The model under review builds one solid part; all positions refer to its coordinate system, in mm. Give positions to 0.01 mm unless a question says otherwise; leave off trailing zeros. Loops run counter-clockwise (first coordinate to the right, second up) from the corner with the lowest first, then second, coordinate; pieces in that order, holes last. Notation, with made-up numbers: M 73,13.25 L 112,13.25 A7 ccw 112,22.25 Z; hole C 40.5,57 d4. An arc over 180 degrees is marked long. Write item = value, one per line. Start each with the question number.
1. We need section B-B on z = 1.5. Count the separate pieces of the cut face and the enclosed holes in it, then the cut area to 3 significant figures.
2. For pin 1 (1.5 mm diameter, centred on x = 66.5, z = 1, fed in from +Y); pin 2 (1.5 mm diameter, centred on y = -84.5, z = 1.5, fed in from +X); pin 3 (0.9 mm diameter, centred on y = 43.5, z = 1, fed in from +X), all flat-tipped, find the tip position at first contact; note any pin that passes through.
3. We need section A-A on x = -4.5. Give the boundary of the cut face in (y, z).
4. We need section C-C on x = -31.5. Give the boundary of the cut face in (y, z), then the cut area to 3 significant figures.
5. Wall thickness on line 1 along X through (y, z) = (-45.5, 1.2); line 2 along Y through (x, z) = (9, 0.35); line 3 along X through (y, z) = (-89, 1.4): over which ranges is each line inside the solid? List them lowest first. Write a range as from..to.
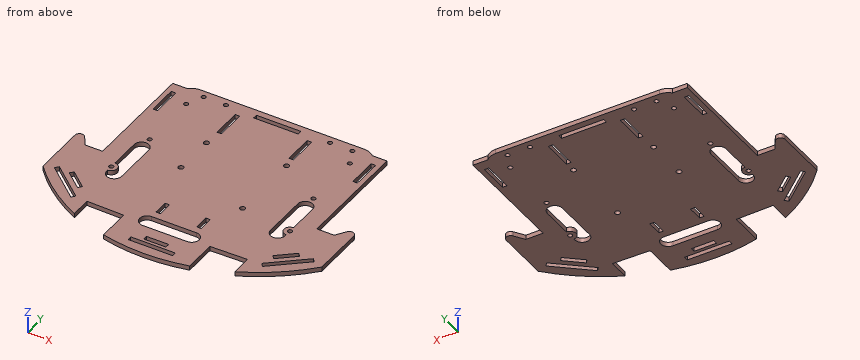
from build123d import *

# Parameters (mm, degrees)
SKETCH1_R           = 1.5
BOSS_EXTRUDE1_DEPTH = 3
SKETCH12_W          = 3
SKETCH12_H          = 20
BOSS_EXTRUDE3_DEPTH = 3
SKETCH13_W          = 3
SKETCH13_H          = 20
CUT_EXTRUDE5_DEPTH  = 3
SKETCH15_W          = 30
SKETCH15_H          = 3
BOSS_EXTRUDE4_DEPTH = 3
CUT_EXTRUDE7_DEPTH  = 3
CUT_EXTRUDE8_DEPTH  = 5
SKETCH18_R          = 1.5
SKETCH18_W          = 30
SKETCH18_H          = 3
CUT_EXTRUDE9_DEPTH  = 3
FILLET4_R           = 3
SKETCH25_R          = 1.5
CUT_EXTRUDE11_DEPTH = 10
CUT_EXTRUDE12_DEPTH = 10
SKETCH27_W          = 15
SKETCH27_H          = 3
CUT_EXTRUDE13_DEPTH = 10
SKETCH34_W          = 3
SKETCH34_H          = 10
CUT_EXTRUDE14_DEPTH = 10
SKETCH35_R          = 1.75
CUT_EXTRUDE15_DEPTH = 10


with BuildPart() as part:
    # Sketch1 → Boss-Extrude1 (new body)
    with BuildSketch(Plane.XY):
        with BuildLine():
            Line((-65, 40), (-65, -45))
            ThreePointArc((-65, -45), (-62.071067812, -52.071067812), (-55, -55))
            Line((-55, -55), (55, -55))
            ThreePointArc((55, -55), (62.071067812, -52.071067812), (65, -45))
            Line((65, -45), (65, 40))
            ThreePointArc((65, 40), (62.071067812, 47.071067812), (55, 50))
            Line((55, 50), (-55, 50))
            ThreePointArc((-55, 50), (-62.071067812, 47.071067812), (-65, 40))
        make_face()
        with Locations((-50, 45)):
            Circle(SKETCH1_R, mode=Mode.SUBTRACT)
        with Locations((50, 45)):
            Circle(SKETCH1_R, mode=Mode.SUBTRACT)
        with Locations((-60, -40)):
            Circle(SKETCH1_R, mode=Mode.SUBTRACT)
        with Locations((60, -40)):
            Circle(SKETCH1_R, mode=Mode.SUBTRACT)
    extrude(amount=BOSS_EXTRUDE1_DEPTH)

    # Sketch12 → Boss-Extrude3 (add)
    with BuildSketch(Plane(origin=(0, 0, 0), x_dir=(-1, 0, 0), z_dir=(0, 0, -1))):
        with BuildLine():
            Line((65, 40), (65, -30))
            Line((65, -30), (72, -30))
            Line((72, -30), (72, 40))
            Line((72, 40), (72, 47.071067812))
            Line((72, 47.071067812), (62.071067812, 47.071067812))
            ThreePointArc((62.071067812, 47.071067812), (64.238795325, 43.826834324), (65, 40))
        make_face()
        with Locations((67.174969976, 30)):
            Rectangle(SKETCH12_W, SKETCH12_H, mode=Mode.SUBTRACT)
        with BuildLine():
            Line((-72, 40), (-72, -30))
            Line((-72, -30), (-65, -30))
            Line((-65, -30), (-65, 40))
            ThreePointArc((-65, 40), (-64.238795325, 43.826834324), (-62.071067812, 47.071067812))
            Line((-62.071067812, 47.071067812), (-72, 47.071067812))
            Line((-72, 47.071067812), (-72, 40))
        make_face()
        with Locations((-67.174969976, 30)):
            Rectangle(SKETCH12_W, SKETCH12_H, mode=Mode.SUBTRACT)
    extrude(amount=-BOSS_EXTRUDE3_DEPTH)

    # Sketch13 → Cut-Extrude5 (cut)
    with BuildSketch(Plane(origin=(0, 0, 0), x_dir=(-1, 0, 0), z_dir=(0, 0, -1))):
        with Locations((24.174969976, 30)):
            Rectangle(SKETCH13_W, SKETCH13_H)
        with Locations((-24.174969976, 30)):
            Rectangle(SKETCH13_W, SKETCH13_H)
    extrude(amount=-CUT_EXTRUDE5_DEPTH, mode=Mode.SUBTRACT)

    # Sketch15 → Boss-Extrude4 (add)
    with BuildSketch(Plane(origin=(0, 0, 0), x_dir=(-1, 0, 0), z_dir=(0, 0, -1))):
        with BuildLine():
            Line((73.674969976, -30), (72, -30))
            Line((72, -30), (65, -30))
            Line((65, -30), (65, -45))
            ThreePointArc((65, -45), (62.071067812, -52.071067812), (55, -55))
            Line((55, -55), (-55, -55))
            ThreePointArc((-55, -55), (-62.071067812, -52.071067812), (-65, -45))
            Line((-65, -45), (-65, -30))
            Line((-65, -30), (-72, -30))
            Line((-72, -30), (-73.674969976, -30))
            Line((-73.674969976, -30), (-83.674969976, -30))
            Line((-83.674969976, -30), (-93.674969976, -15))
            Line((-93.674969976, -15), (-93.674969976, -60))
            ThreePointArc((-93.674969976, -60), (-75.11867005, -76.957696294), (-53.544667826, -89.859717787))
            Line((-53.544667826, -89.859717787), (-53.544667826, -77.921197712))
            Line((-53.544667826, -77.921197712), (-43.544667826, -77.921197712))
            Line((-43.544667826, -77.921197712), (-28.544667826, -78.447755309))
            Line((-28.544667826, -78.447755309), (-28.544667826, -98.657929362))
            ThreePointArc((-28.544667826, -98.657929362), (0.412515012, -102.058251887), (29.36969785, -98.657929362))
            Line((29.36969785, -98.657929362), (29.36969785, -78.447755309))
            Line((29.36969785, -78.447755309), (44.36969785, -77.921197712))
            Line((44.36969785, -77.921197712), (54.36969785, -77.921197712))
            Line((54.36969785, -77.921197712), (54.36969785, -89.791641118))
            ThreePointArc((54.36969785, -89.791641118), (75.506234101, -76.853587855), (93.674969976, -60))
            Line((93.674969976, -60), (93.674969976, -15))
            Line((93.674969976, -15), (83.674969976, -30))
            Line((83.674969976, -30), (73.674969976, -30))
        make_face()
        Polygon((-64.364341028, -77.265224848), (-87.294606331, -57.920899244), (-85.360173771, -55.627872713), (-62.429908467, -74.972198318), align=None, mode=Mode.SUBTRACT)
        with Locations((0, -93.735273214)):
            Rectangle(SKETCH15_W, SKETCH15_H, mode=Mode.SUBTRACT)
        Polygon((-65.960254421, -67.497898332), (-77.422828052, -57.822702946), (-75.487788974, -55.53018822), (-64.025215344, -65.205383606), align=None, mode=Mode.SUBTRACT)
        Polygon((85.360173771, -55.627872713), (87.294606331, -57.920899244), (64.364341028, -77.265224848), (62.429908467, -74.972198318), align=None, mode=Mode.SUBTRACT)
        Polygon((77.394030345, -57.788043022), (65.932380202, -67.464332393), (63.997122328, -65.172002365), (75.458772471, -55.495712994), align=None, mode=Mode.SUBTRACT)
    extrude(amount=-BOSS_EXTRUDE4_DEPTH)

    # Sketch16 → Cut-Extrude7 (cut)
    with BuildSketch(Plane(origin=(0, 0, 0), x_dir=(-1, 0, 0), z_dir=(0, 0, -1))):
        with BuildLine():
            Line((-60, -44), (-60, -45))
            ThreePointArc((-60, -45), (-55, -50), (-50, -45))
            Line((-50, -45), (-50, -15))
            ThreePointArc((-50, -15), (-55, -10), (-60, -15))
            Line((-60, -15), (-60, -36))
            ThreePointArc((-60, -36), (-56, -40), (-60, -44))
        make_face()
        with BuildLine():
            Line((60, -36), (60, -15))
            ThreePointArc((60, -15), (55, -10), (50, -15))
            Line((50, -15), (50, -45))
            ThreePointArc((50, -45), (55, -50), (60, -45))
            Line((60, -45), (60, -44))
            ThreePointArc((60, -44), (56, -40), (60, -36))
        make_face()
    extrude(amount=-CUT_EXTRUDE7_DEPTH, mode=Mode.SUBTRACT)

    # Sketch17 → Cut-Extrude8 (cut)
    with BuildSketch(Plane(origin=(0, 0, 0), x_dir=(-1, 0, 0), z_dir=(0, 0, -1))):
        with BuildLine():
            Line((-15, -69.235273214), (15, -69.235273214))
            ThreePointArc((15, -69.235273214), (20, -74.235273214), (15, -79.235273214))
            Line((15, -79.235273214), (-15, -79.235273214))
            ThreePointArc((-15, -79.235273214), (-20, -74.235273214), (-15, -69.235273214))
        make_face()
    extrude(amount=-CUT_EXTRUDE8_DEPTH, mode=Mode.SUBTRACT)

    # Sketch18 → Cut-Extrude9 (cut)
    with BuildSketch(Plane(origin=(0, 0, 0), x_dir=(-1, 0, 0), z_dir=(0, 0, -1))):
        with Locations((55, 34)):
            Circle(SKETCH18_R)
        with Locations((55, -6)):
            Circle(SKETCH18_R)
        with Locations((-55, 34)):
            Circle(SKETCH18_R)
        with Locations((-55, -6)):
            Circle(SKETCH18_R)
        with Locations((0, 44.264726786)):
            Rectangle(SKETCH18_W, SKETCH18_H)
    extrude(amount=-CUT_EXTRUDE9_DEPTH, mode=Mode.SUBTRACT)

    # Fillet4
    fillet4_edges = [part.edges().sort_by_distance(p)[0] for p in [
        (93.674969976, -15, 1.5),
        (-93.674969976, -15, 1.5),
    ]]
    fillet(fillet4_edges, radius=FILLET4_R)

    # Sketch25 → Cut-Extrude11 (cut)
    with BuildSketch(Plane.XY.offset(3)):
        with Locations((-35, 45)):
            Circle(SKETCH25_R)
        with Locations((35, 45)):
            Circle(SKETCH25_R)
    extrude(amount=-CUT_EXTRUDE11_DEPTH, mode=Mode.SUBTRACT)

    # Sketch26 → Cut-Extrude12 (cut)
    with BuildSketch(Plane.XY.offset(3)):
        Polygon((-54.36969785, -77.921197712), (-54.36969785, -75.921197712), (-29.36969785, -76.450833315), (-29.36969785, -78.447755309), align=None)
        Polygon((28.544667826, -78.447755309), (28.544667826, -76.450833315), (53.544667826, -75.921197712), (53.544667826, -77.921197712), align=None)
    extrude(amount=-CUT_EXTRUDE12_DEPTH, mode=Mode.SUBTRACT)

    # Sketch27 → Cut-Extrude13 (cut)
    with BuildSketch(Plane(origin=(0, 0, 0), x_dir=(-1, 0, 0), z_dir=(0, 0, -1))):
        with Locations((0.14797788, -88.645273214)):
            Rectangle(SKETCH27_W, SKETCH27_H)
    extrude(amount=-CUT_EXTRUDE13_DEPTH, mode=Mode.SUBTRACT)

    # Sketch34 → Cut-Extrude14 (cut)
    with BuildSketch(Plane.XY.offset(3)):
        with Locations((13.7, -59.235273214)):
            Rectangle(SKETCH34_W, SKETCH34_H)
        with Locations((-13.7, -59.235273214)):
            Rectangle(SKETCH34_W, SKETCH34_H)
    extrude(amount=-CUT_EXTRUDE14_DEPTH, mode=Mode.SUBTRACT)

    # Sketch35 → Cut-Extrude15 (cut)
    with BuildSketch(Plane.XY.offset(3)):
        with Locations((25.3, -35.3)):
            Circle(SKETCH35_R)
        with Locations((-25.5, -19.9)):
            Circle(SKETCH35_R)
        with Locations((25.3, 13)):
            Circle(SKETCH35_R)
        with Locations((-25.5, 8)):
            Circle(SKETCH35_R)
    extrude(amount=-CUT_EXTRUDE15_DEPTH, mode=Mode.SUBTRACT)


solid = part.part
Final values:
q1.separate_pieces = 1
q1.enclosed_holes = 30
q1.area = 19,700 mm²
q2.pin_1 = 47.07
q2.pin_2 = 64.99
q2.pin_3 = 72
q3.outline = M -101.99,0 L -95.24,0 L -95.24,3 L -101.99,3 Z; M -92.24,0 L -90.15,0 L -90.15,3 L -92.24,3 Z; M -87.15,0 L -79.24,0 L -79.24,3 L -87.15,3 Z; M -69.24,0 L 42.76,0 L 42.76,3 L -69.24,3 Z; M 45.76,0 L 50,0 L 50,3 L 45.76,3 Z
q4.outline = M -76.41,0 L 50,0 L 50,3 L -76.41,3 Z
q4.area = 379 mm²
q5.line_1 = -93.67..-59.97, -50.03..50.03, 59.97..93.67
q5.line_2 = -101.7..-95.24, -92.24..-79.24, -69.24..42.76, 45.76..50
q5.line_3 = -55.98..-54.37, -29.37..-7.65, 7.35..28.54, 53.54..55.34
